```python
from build123d import *

# Parameters (mm, degrees)
BOSS_EXTRUDE1_DEPTH  = 5
BOSS_EXTRUDE2_DEPTH  = 10
SKETCH3_R            = 2.54
CUT_EXTRUDE1_DEPTH   = 115.031574575
SKETCH5_W            = 13.851899184
SKETCH5_H            = 25.842671822
BOSS_EXTRUDE3_DEPTH  = 2.54
SKETCH6_W            = 9.079065489
SKETCH6_H            = 2.54
BOSS_EXTRUDE7_DEPTH  = 25.4
SKETCH9_R            = 24.13
BOSS_EXTRUDE10_DEPTH = 12.7
SKETCH12_W           = 9.079065489
SKETCH12_H           = 25.611184956
BOSS_EXTRUDE11_DEPTH = 2.54


with BuildPart() as part:
    # Sketch1 → Boss-Extrude1 (new body)
    with BuildSketch(Plane(origin=(0, 0, 0), x_dir=(1, 0, 0), z_dir=(0, 1, 0))):
        Polygon((101.6, 50.8), (88.9, 50.8), (88.9, 38.1), (-17.78, 38.1), (-17.78, 50.8), (-101.6, 50.8), (-101.6, -50.8), (-17.78, -50.8), (-17.78, -38.1), (88.9, -38.1), (88.9, -50.8), (101.6, -50.8), align=None)
    extrude(amount=BOSS_EXTRUDE1_DEPTH)

    # Sketch2 → Boss-Extrude2 (add)
    with BuildSketch(Plane(origin=(0, 5, 0), x_dir=(1, 0, 0), z_dir=(0, 1, 0))):
        Polygon((88.9, -38.1), (88.9, -20.32), (-17.78, -20.32), (-17.78, -17.78), (91.44, -17.78), (91.44, -38.1), align=None)
        Polygon((91.44, 17.78), (91.44, 38.1), (88.9, 38.1), (88.9, 20.32), (-17.78, 20.32), (-17.78, 17.78), align=None)
    extrude(amount=BOSS_EXTRUDE2_DEPTH)

    # Sketch3 → Cut-Extrude1 (cut, through all)
    with BuildSketch(Plane(origin=(0, 5, 0), x_dir=(1, 0, 0), z_dir=(0, 1, 0))):
        with Locations(Location((-25.086891482, 28.312348959, 0), (0, 0, 270))):
            Circle(SKETCH3_R)
        with Locations(Location((-25.086891482, -28.312348959, 0), (0, 0, 90))):
            Circle(SKETCH3_R)
    extrude(amount=-CUT_EXTRUDE1_DEPTH, mode=Mode.SUBTRACT)

    # Sketch5 → Boss-Extrude3 (add)
    with BuildSketch(Plane(origin=(0, 5, 0), x_dir=(1, 0, 0), z_dir=(0, 1, 0))):
        with Locations((-59.69, 0)):
            Rectangle(SKETCH5_W, SKETCH5_H)
    extrude(amount=BOSS_EXTRUDE3_DEPTH)

    # Sketch6 → Boss-Extrude7 (add)
    with BuildSketch(Plane(origin=(0, 7.54, 0), x_dir=(1, 0, 0), z_dir=(0, 1, 0))):
        with Locations((-59.730694006, 7.841335911)):
            Rectangle(SKETCH6_W, SKETCH6_H)
    extrude(amount=BOSS_EXTRUDE7_DEPTH)

    # Sketch9 → Boss-Extrude10 (add)
    with BuildSketch(Plane.XY.offset(-6.571335911)):
        with Locations(Location((-59.730694006, 32.94, 0), (0, 0, 259.156433542))):
            Circle(SKETCH9_R)
    extrude(amount=BOSS_EXTRUDE10_DEPTH)

    # Sketch12 → Boss-Extrude11 (add)
    with BuildSketch(Plane.XY.offset(6.128664089)):
        with Locations((-59.730694006, 20.134407522)):
            Rectangle(SKETCH12_W, SKETCH12_H)
    extrude(amount=BOSS_EXTRUDE11_DEPTH)


solid = part.part
```
Input: part model. Units: mm. Frame: model coordinates. A direction names the side the tool comes from. Give positions to 0.01 mm unless a question says otherwise; leave off trailing zeros. Order: outer loops, then holes, each group sorted by start corner. A loop starts at its lowest first (then second) coordinate and runs counter-clockwise, first axis right, second up. Notation, with made-up numbers: (69.5, 88.25) - (86.5, 88.25) arc R30 ccw to (86.5, 122.25) - close; hole circle Ø1 at (66, -14.5). An arc over 180 degrees is marked (long way). Use a Markdown table: item, result.
(1) Draft query along X for faces 4 (the flat face through (91.44, 10, 28)), 5 (the cylindrical face through (-25.85, 2.54, 25.89)), 6 (the flat face through (-59, 2, -50.8)). Return one class per face: released by +X, released by -X, zero draft, split by the parting line, or undercut.
Computed values:
| item | result |
|---|---|
| face 4 | released by +X |
| face 5 | undercut |
| face 6 | zero draft |
(2) Section query B-B (x = 37.5). Output: boundary loops of the cut face in (y, z), then the cut area to 3 significant figures.
Computed values:
| item | result |
|---|---|
| outline | (0, -38.1) - (5, -38.1) - (5, -20.32) - (15, -20.32) - (15, -17.78) - (5, -17.78) - (5, 17.78) - (15, 17.78) - (15, 20.32) - (5, 20.32) - (5, 38.1) - (0, 38.1) - close |
| area | 432 mm2 |
(3) Access query for faces 1 (the flat face through (-60, 20, 8.669)), 2 (the flat face through (-60, 20, -9.111)), 3 (the flat face through (36, 10, -17.78)). Directions: +Z, -Z, +X, -X, +Y, -Y. A direction counts if a zero-diameter tool reaches every point of the face in a straight line with its end or side. Return the directions, or none.
Computed values:
| item | result |
|---|---|
| face 1 | +Z, +X, -X, +Y |
| face 2 | -Z, +X, -X, +Y |
| face 3 | +X, -X, +Y |
(4) Section query A-A (z = 3.5). Output: boundary loops of the cut face in (x, y), then the cut area to 3 significant figures.
Computed values:
| item | result |
|---|---|
| outline | (-101.6, 0) - (101.6, 0) - (101.6, 5) - (-52.76, 5) - (-52.76, 7.54) - (-66.62, 7.54) - (-66.62, 5) - (-101.6, 5) - close; circle Ø48.26 at (-59.73, 32.94) |
| area | 2,880 mm2 |
(5) Section query D-D (y = 45). Output: boundary loops of the cut face in (x, z), then the cut area to 3 significant figures.
Computed values:
| item | result |
|---|---|
| outline | (-80.63, -6.57) - (-38.83, -6.57) - (-38.83, 6.13) - (-80.63, 6.13) - close |
| area | 531 mm2 |
(6) Section query C-C (y = 23). Output: boundary loops of the cut face in (x, z).
Computed values:
| item | result |
|---|---|
| outline | (-81.72, -6.57) - (-64.27, -6.57) - (-64.27, -9.11) - (-55.19, -9.11) - (-55.19, -6.57) - (-37.74, -6.57) - (-37.74, 6.13) - (-55.19, 6.13) - (-55.19, 8.67) - (-64.27, 8.67) - (-64.27, 6.13) - (-81.72, 6.13) - close |
(7) Line query: line 1 (Y direction, x = 9, z = 3.5); line 2 (Z direction, x = -7, y = 4); line 3 (Z direction, x = -49.5, y = 33). Output: solid intervals per line, ascending. Write a range as from..to.
Computed values:
| item | result |
|---|---|
| line 1 | y = 0..5 |
| line 2 | z = -38.1..38.1 |
| line 3 | z = -6.57..6.13 |
(8) Pin query (flat end, axial travel): pin 1 (3 mm diameter, centred on y = 14, z = 8, fed in from +X); pin 2 (3 mm diameter, centred on y = 9.5, z = -25.5, fed in from -X); pin 3 (2 mm diameter, centred on x = 90.5, y = 10.5, fed in from -Z); pin 4 (4 mm diameter, centred on x = -25.09, z = 28.31, fed in from +Y). Return the tip coordinate at first contact, or that it passes through.
Computed values:
| item | result |
|---|---|
| pin 1 | stops at x = -55.19 |
| pin 2 | stops at x = 88.9 |
| pin 3 | stops at z = -38.1 |
| pin 4 | passes through |
